Here's how the part is built. I have some questions about the finished solid (model axes, mm). Face numbers are marked on the shaded views. Round coordinates to 2 decimals unless told otherwise and drop trailing zeros. Write each loop counter-clockwise with the first axis right and the second up, starting at its lowest first coordinate (ties: lowest second). Pieces come first, ordered by that corner, then holes. Notation, with made-up numbers: (26.5, 80.25) -> (31.5, 80.25) arc R21 cw to (31.5, 89.25) -> close; hole circle Ø6 at (-35, 77.5). An arc over 180 degrees is marked (long way). Answer in a Markdown table with one row per item. Add a question column.
from build123d import *

# Parameters (mm, degrees)
SKETCH1_R           = 3.175
BOSS_EXTRUDE1_DEPTH = 6.35
SKETCH2_R           = 1.016
CUT_EXTRUDE1_DEPTH  = 9.144


with BuildPart() as part:
    # Sketch1 → Boss-Extrude1 (new body)
    with BuildSketch(Plane.XY):
        with BuildLine():
            Line((-5.715, -9.525), (5.715, -9.525))
            Line((5.715, -9.525), (5.715, 0))
            ThreePointArc((5.715, 0), (0, 5.715), (-5.715, 0))
            Line((-5.715, 0), (-5.715, -9.525))
        make_face()
        Circle(SKETCH1_R, mode=Mode.SUBTRACT)
    extrude(amount=BOSS_EXTRUDE1_DEPTH)

    # Sketch2 → Cut-Extrude1 (cut)
    with BuildSketch(Plane.XZ.offset(9.525)):
        with Locations((0, 3.175)):
            Circle(SKETCH2_R)
    extrude(amount=-CUT_EXTRUDE1_DEPTH, mode=Mode.SUBTRACT)


solid = part.part
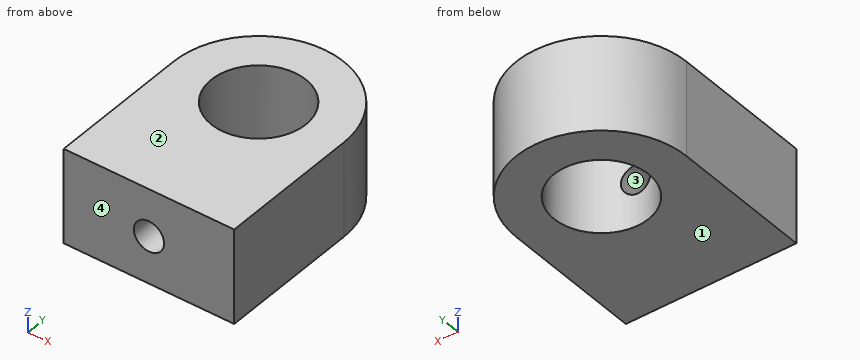
Item 1: If we section it at A-A on x = 0: Please give me the cut outline in (y, z) (3 decimals), then the cut area to 3 significant figures.
Item 2: If we mould it in two halves opening along Z, with no side actions, what happens to the marked faces 1, 2, 3 and 4? For each: pulls with the +Z half, pulls with the -Z half, needs draft (parallel to the pull), parting line crosses it, or undercut.
Item 3: If we section it at C-C on y = -0.5: Please give me the cut outline in (x, z) (3 decimals).
Item 4: If we section it at D-D on x = -2: Please give me the cut outline in (y, z) (3 decimals).
Item 5: I need wall thicknesses on line 1 along Z through (x, y) = (0, -6.5); line 2 along X through (y, z) = (-8.5, 3.25) (3 decimals); line 3 along Y through (x, z) = (0, 3.25) (3 decimals). Which ranges of each line are inside material? Lowest first, please. Write a range as from..to.
Item 6: If we section it at B-B on z = 0.5: Please give me the cut outline in (x, y) (3 decimals), then the cut area to 3 significant figures.
Item 7: For P1, Ø3, axis at x = 3.5, z = 4, coming from the +Y side, with a flat end and sliding along its axis, tell me the tip position at first contact or that it passes through.
Results list:
| question | item | result |
|---|---|---|
| 1 | outline | (-9.525, 0) -> (-3.175, 0) -> (-3.175, 2.159) -> (-9.525, 2.159) -> close; (-9.525, 4.191) -> (-3.175, 4.191) -> (-3.175, 6.35) -> (-9.525, 6.35) -> close; (3.175, 0) -> (5.715, 0) -> (5.715, 6.35) -> (3.175, 6.35) -> close |
| 1 | area | 43.5 mm² |
| 2 | face 1 | pulls with the -Z half |
| 2 | face 2 | pulls with the +Z half |
| 2 | face 3 | undercut |
| 2 | face 4 | needs draft |
| 3 | outline | (-5.715, 0) -> (-3.135, 0) -> (-3.135, 6.35) -> (-5.715, 6.35) -> close; (3.135, 0) -> (5.715, 0) -> (5.715, 6.35) -> (3.135, 6.35) -> close |
| 4 | outline | (-9.525, 0) -> (-2.466, 0) -> (-2.466, 6.35) -> (-9.525, 6.35) -> close; (2.466, 0) -> (5.354, 0) -> (5.354, 6.35) -> (2.466, 6.35) -> close |
| 5 | line 1 | 0..2.16, 4.19..6.35 |
| 5 | line 2 | -5.715..-1.013, 1.013..5.715 |
| 5 | line 3 | 3.175..5.715 |
| 6 | outline | (-5.715, -9.525) -> (5.715, -9.525) -> (5.715, 0) arc R5.715 ccw to (-5.715, 0) -> close; hole circle Ø6.35 at (0, 0) |
| 6 | area | 129 mm² |
| 7 | P1 | y = 5.35 |
